CAD build for the part. Positions are in the model's coordinates, mm. A direction names the side the tool comes from. Give positions to 0.01 mm unless a question says otherwise; leave off trailing zeros. Write each loop counter-clockwise with the first axis right and the second up, starting at its lowest first coordinate (ties: lowest second). Pieces come first, ordered by that corner, then holes. Notation, with made-up numbers: (76, 84.25) -> (93, 84.25) arc R36 ccw to (93, 119.25) -> close; hole circle Ø9 at (-37.5, 64.5). An arc over 180 degrees is marked (long way). Answer as a JSON object with one key per item and string values.
```python
from build123d import *

# Parameters (mm, degrees)
BOSS_EXTRUDE1_DEPTH = 10
SKETCH2_R           = 9
BOSS_EXTRUDE2_DEPTH = 10
BOSS_EXTRUDE3_DEPTH = 10
SKETCH4_W           = 55
SKETCH4_H           = 60
BOSS_EXTRUDE4_DEPTH = 10
SKETCH5_R           = 9
CUT_EXTRUDE1_DEPTH  = 38


with BuildPart() as part:
    # Sketch1 → Boss-Extrude1 (new body)
    with BuildSketch(Plane(origin=(0, 0, 0), x_dir=(1, 0, 0), z_dir=(0, 1, 0))):
        with BuildLine():
            Line((0, -36.704850043), (55, -36.704850043))
            Line((55, -36.704850043), (55, 23.295149957))
            Line((55, 23.295149957), (-85, 23.295149957))
            ThreePointArc((-85, 23.295149957), (-92.071067812, 20.366217769), (-95, 13.295149957))
            Line((-95, 13.295149957), (-95, -6.704850043))
            Line((-95, -6.704850043), (-88.5, -6.704850043))
            Line((-88.5, -6.704850043), (-88.5, 3.295149957))
            ThreePointArc((-88.5, 3.295149957), (-82.5, 9.295149957), (-76.5, 3.295149957))
            Line((-76.5, 3.295149957), (-76.5, -6.704850043))
            Line((-76.5, -6.704850043), (-70, -6.704850043))
            Line((-70, -6.704850043), (-70, -2.704850043))
            Line((-70, -2.704850043), (0, -36.704850043))
        make_face()
    extrude(amount=BOSS_EXTRUDE1_DEPTH)

    # Sketch2 → Boss-Extrude2 (add)
    with BuildSketch(Plane.ZY.offset(-55)):
        with BuildLine():
            Line((-23.295149957, 10), (36.704850043, 10))
            Line((36.704850043, 10), (36.704850043, 18))
            ThreePointArc((36.704850043, 18), (52.704850043, 34), (36.704850043, 50))
            Line((36.704850043, 50), (-23.295149957, 50))
            Line((-23.295149957, 50), (-23.295149957, 10))
        make_face()
        with Locations((36.704850043, 34)):
            Circle(SKETCH2_R, mode=Mode.SUBTRACT)
    extrude(amount=BOSS_EXTRUDE2_DEPTH)

    # Sketch3 → Boss-Extrude3 (add)
    with BuildSketch(Plane.XY.offset(-23.295149957)):
        Polygon((45, 10), (-70, 10), (10, 50), (45, 50), (45, 11.165402215), align=None)
    extrude(amount=BOSS_EXTRUDE3_DEPTH)

    # Sketch4 → Boss-Extrude4 (add)
    with BuildSketch(Plane(origin=(0, 0, 0), x_dir=(-1, 0, 0), z_dir=(0, -1, 0))):
        with Locations((-27.5, -6.704850043)):
            Rectangle(SKETCH4_W, SKETCH4_H)
    extrude(amount=BOSS_EXTRUDE4_DEPTH)

    # Sketch5 → Cut-Extrude1 (cut)
    with BuildSketch(Plane(origin=(0, 10, 0), x_dir=(1, 0, 0), z_dir=(0, 1, 0))):
        with Locations(Location((30, -11.704850043, 0), (0, 0, 270))):
            Circle(SKETCH5_R)
    extrude(amount=-CUT_EXTRUDE1_DEPTH, mode=Mode.SUBTRACT)


solid = part.part
```
1) Slice it at A-A (y = 8). List the corners of the cut face in (x, z), then the cut area to 3 significant figures.
Model answer:
{"outline": "(-95, -13.3) arc R10 ccw to (-85, -23.3) -> (55, -23.3) -> (55, 36.7) -> (0, 36.7) -> (-70, 2.7) -> (-70, 6.7) -> (-76.5, 6.7) -> (-76.5, -3.3) arc R6 cw to (-88.5, -3.3) -> (-88.5, 6.7) -> (-95, 6.7) -> close; hole circle Ø18 at (30, 11.7)", "area": "6,610 mm2"}
2) Slice it at C-C (y = 34). List the corners of the cut face in (x, z), then the cut area to 3 significant figures.
Model answer:
{"outline": "(-22, -23.3) -> (55, -23.3) -> (55, 27.7) -> (45, 27.7) -> (45, -13.3) -> (-22, -13.3) -> close; (45, 45.7) -> (55, 45.7) -> (55, 52.7) -> (45, 52.7) -> close", "area": "1,250 mm2"}
3) Pin check, flat tips, straight feed: pin 1 (5 mm diameter, centred on x = -72, y = 4.5, fed in from +Z); pin 2 (2 mm diameter, centred on y = 37, z = 8, fed in from -X); pin 3 (1.5 mm diameter, centred on x = 22, z = 19.5, fed in from +Y). Stop position of each tip, or through.
Model answer:
{"pin 1": "stops at z = 6.7", "pin 2": "stops at x = 45", "pin 3": "stops at y = 10"}
4) Wall check: probe 1 along X at (y, z) = (-2, 11); probe 2 along Y at (x, z) = (16, -9); probe 3 along Y at (x, z) = (-85.5, -15). Give the ranges that are in metal, low to high.
Model answer:
{"probe 1": "x = 0 to 21.03, 38.97 to 55", "probe 2": "y = -10 to 10", "probe 3": "y = 0 to 10"}
5) 3-axis set-ups, long thin cutter, end or side, ignore diameter. For faces 1 (the flat face through (-10, 10, 6)), 2 (the flat face through (-73, 5, 6.705)), 3 (the flat face through (28, 1, 36.705)): which of +Z, -Z, +X, -X, +Y, -Y reach the whole face in a straight line?
Model answer:
{"face 1": "+Z, -X, +Y", "face 2": "+Z, -X, +Y, -Y", "face 3": "+Z, +X, -X, -Y"}
6) Slice it at D-D (z = 40). List the corners of the cut face in (x, y), then the cut area to 3 significant figures.
Model answer:
{"outline": "(45, 18.34) -> (55, 18.34) -> (55, 25.62) -> (45, 25.62) -> close; (45, 42.38) -> (55, 42.38) -> (55, 49.66) -> (45, 49.66) -> close", "area": "146 mm2"}
7) Mould opens along Z. For faces 4 (the flat face through (-92, 5, 6.705)), 5 (the cylindrical face through (50.07, 42.923, 35.533)), 6 (the flat face through (22, -10, 6)) say: released by +Z, released by -Z, zero draft, split by the parting line, or undercut.
Model answer:
{"face 4": "released by +Z", "face 5": "undercut", "face 6": "zero draft"}
8) Slice it at B-B (x = 30). List the corners of the cut face in (y, z).
Model answer:
{"outline": "(-10, -23.3) -> (50, -23.3) -> (50, -13.3) -> (10, -13.3) -> (10, 2.7) -> (-10, 2.7) -> close; (-10, 20.7) -> (10, 20.7) -> (10, 36.7) -> (-10, 36.7) -> close"}
